```python
from build123d import *

# Parameters (mm, degrees)
CROQUIS1_W                 = 25.4
CROQUIS1_H                 = 25.4
SALIENTE_EXTRUIR1_DEPTH    = 40
SALIENTE_EXTRUIR3_DEPTH    = 17.5
SALIENTE_EXTRUIR4_REACH    = 76.655
CROQUIS6_W                 = 10
CROQUIS6_H                 = 20
CROQUIS9_R                 = 3.25
CORTAR_EXTRUIR3_DEPTH      = 10
CORTAR_EXTRUIR4_START      = -2.5
CROQUIS10_W                = 6.5
CROQUIS10_H                = 6.5
CORTAR_EXTRUIR4_DEPTH      = 10
CORTAR_EXTRUIR1_DEPTH      = 67.880303528
CORTAR_EXTRUIR1_DEPTH_BACK = 67.880303528
CROQUIS7_R                 = 3.5
SALIENTE_EXTRUIR5_START    = 21
CROQUIS11_W                = 10
CROQUIS11_H                = 10
CROQUIS11_R                = 3.5
SALIENTE_EXTRUIR5_DEPTH    = 21
SALIENTE_EXTRUIR6_START    = -10
SALIENTE_EXTRUIR6_DEPTH    = 10


with BuildPart() as part:
    # Croquis1 → Saliente-Extruir1 (new body)
    with BuildSketch(Plane(origin=(0, 0, 0), x_dir=(1, 0, 0), z_dir=(0, 1, 0))):
        Rectangle(CROQUIS1_W, CROQUIS1_H)
        Polygon((-10.2, 10.2), (-2.5, 10.2), (-2.5, 5.2), (2.5, 5.2), (2.5, 10.2), (10.2, 10.2), (10.2, 2.5), (5.2, 2.5), (5.2, -2.5), (10.2, -2.5), (10.2, -10.2), (2.5, -10.2), (2.5, -5.2), (-2.5, -5.2), (-2.5, -10.2), (-10.2, -10.2), (-10.2, -2.5), (-5.2, -2.5), (-5.2, 2.5), (-10.2, 2.5), align=None, mode=Mode.SUBTRACT)
    extrude(amount=SALIENTE_EXTRUIR1_DEPTH)



with BuildPart() as body_2:
    # Croquis4 → Saliente-Extruir3 (new, symmetric)
    with BuildSketch(Plane.XY):
        Polygon((-52.043145751, 35.556349186), (-47.093398282, 30.606601718), (-68.306601718, 9.393398282), (-73.256349186, 14.343145751), align=None)
    extrude(amount=SALIENTE_EXTRUIR3_DEPTH, both=True)


with BuildPart() as part_1:
    add(part.part)

    add(body_2.part)  # Saliente-Extruir4 merges body 2
    # Saliente-Extruir4: up to this plane
    saliente_extruir4_end = Plane(origin=(-68.306601718, 9.393398282, 17.5), z_dir=(-0.7071067811865436, 0.7071067811865516, 0))
    # Croquis6 → Saliente-Extruir4 (add, up to the surface)
    with BuildSketch(Plane.ZY.offset(12.7), mode=Mode.PRIVATE) as saliente_extruir4_sk1:
        with Locations((0, 20)):
            Rectangle(CROQUIS6_W, CROQUIS6_H)
    saliente_extruir4_tool1 = split(extrude(saliente_extruir4_sk1.sketch, amount=SALIENTE_EXTRUIR4_REACH, mode=Mode.PRIVATE), bisect_by=saliente_extruir4_end, keep=Keep.BOTH, mode=Mode.PRIVATE)
    add(saliente_extruir4_tool1.solids().sort_by_distance((-12.7, 20, 0))[0])

    # Croquis9 → Cortar-Extruir3 (cut)
    with BuildSketch(Plane(origin=(12.7, 0, 0), x_dir=(0, 0, -1), z_dir=(1, 0, 0))):
        with Locations((0, 20)):
            Circle(CROQUIS9_R)
    extrude(amount=-CORTAR_EXTRUIR3_DEPTH, mode=Mode.SUBTRACT)

    # Croquis10 → Cortar-Extruir4 (cut)
    with BuildSketch(Plane(origin=(12.7, 0, 0), x_dir=(0, 0, -1), z_dir=(1, 0, 0)).offset(CORTAR_EXTRUIR4_START)):
        with Locations((0, 20)):
            Rectangle(CROQUIS10_W, CROQUIS10_H)
    extrude(amount=-CORTAR_EXTRUIR4_DEPTH, mode=Mode.SUBTRACT)

    # Croquis7 → Cortar-Extruir1 (cut, two sides: drawn at the far end of the back side and taken through both)
    with BuildSketch(Plane(origin=(-38.85, 38.85, 0), x_dir=(0, 0, -1), z_dir=(0.7071067811865438, -0.7071067811865512, 0)).offset(-CORTAR_EXTRUIR1_DEPTH_BACK)):
        with Locations(Location((0, -26.657925651, 0), (0, 0, 90))):
            Circle(CROQUIS7_R)
    extrude(amount=CORTAR_EXTRUIR1_DEPTH + CORTAR_EXTRUIR1_DEPTH_BACK, mode=Mode.SUBTRACT)

    # Croquis11 → Saliente-Extruir5 (add)
    with BuildSketch(Plane(origin=(-38.85, 38.85, 0), x_dir=(0, 0, -1), z_dir=(0.7071067811865437, -0.7071067811865515, 0)).offset(SALIENTE_EXTRUIR5_START)):
        with Locations((0, -26.657925651)):
            Rectangle(CROQUIS11_W, CROQUIS11_H)
        with Locations(Location((0, -26.657925651, 0), (0, 0, 90))):
            Circle(CROQUIS11_R, mode=Mode.SUBTRACT)
    extrude(amount=-SALIENTE_EXTRUIR5_DEPTH)

    # Croquis12 → Saliente-Extruir6 (add)
    with BuildSketch(Plane.XY.offset(5).offset(SALIENTE_EXTRUIR6_START)):
        Polygon((-38.00151519, 10), (-40.628932188, 10), (-39.315223689, 8.686291501), align=None)
    extrude(amount=SALIENTE_EXTRUIR6_DEPTH)


solid = part_1.part
```
Source: CAD feature listing. Evaluate the final solid. Frame: model axes, mm. A direction names the side the tool comes from. Coordinates: 2 decimals unless noted, no trailing zeros. Write each loop counter-clockwise with the first axis right and the second up, starting at its lowest first coordinate (ties: lowest second). Pieces come first, ordered by that corner, then holes. Notation, with made-up numbers: M 23,88 L 77,88 A16 cw 77,105 Z; hole C 87,3 d8. An arc over 180 degrees is marked long. Answer as a JSON object with one key per item and string values.
1. Cut plane C-C on x = -23. Output: boundary loops of the cut face in (y, z).
Evaluation:
{"outline": "M 10,-5 L 30,-5 L 30,5 L 10,5 Z"}
2. Contact query for flat-ended pins moving along their axis: P1, Ø2, axis at x = -6.5, y = 22.5, coming from the +Z side; P2, Ø1.5, axis at x = 0.5, y = 10.5, coming from the -Z side; P3, Ø2.5, axis at y = 29.5, z = 1, coming from the -X side; P4, Ø10, axis at x = -31, z = -12, coming from the +Y side. Output: stop coordinate, or through.
Evaluation:
{"P1": "z = 12.7", "P2": "z = -12.7", "P3": "x = -59.35", "P4": "through"}
3. Cut plane A-A on z = 8.5. Output: boundary loops of the cut face in (x, y).
Evaluation:
{"outline": "M -73.26,14.34 L -68.31,9.39 L -47.09,30.61 L -52.04,35.56 Z; M -12.7,0 L -10.2,0 L -10.2,40 L -12.7,40 Z; M -2.5,0 L 2.5,0 L 2.5,40 L -2.5,40 Z; M 10.2,0 L 12.7,0 L 12.7,40 L 10.2,40 Z"}
4. Cut plane D-D on z = 1.5. State how many separate pieces and enclosed holes the cut face has, plus the area to 3 significant figures.
Evaluation:
{"separate pieces": "4", "enclosed holes": "0", "area": "1,560 mm^2"}
5. Access query for faces 1 (the flat face through (-62.8, 24.8, 4.1)), 2 (the flat face through (-61, 22, -17.5)), 3 (the flat face through (8, 23.25, 0)), 4 (the flat face through (-40, 8, -1)), 5 (the flat face through (-2.5, 20, 8)). Directions: +Z, -Z, +X, -X, +Y, -Y. A direction counts if a zero-diameter tool reaches every point of the face in a straight line with its end or side. Return the directions, or none.
Evaluation:
{"face 1": "+Z, -Z, -X, +Y", "face 2": "-Z, +X, -X, +Y, -Y", "face 3": "none", "face 4": "+Z, -Z, -Y", "face 5": "+Y, -Y"}
6. Ray query, L1, parallel to Z at x = 10.75, y = 20; L2, parallel to Y at x = 11.65, z = 0; L3, parallel to Z at x = -1.5, y = 19. Return the intervals inside material, ascending.
Evaluation:
{"L1": "-12.7 to -3.25, 3.25 to 12.7", "L2": "0 to 16.75, 23.25 to 40", "L3": "-12.7 to -5.2, 5.2 to 12.7"}
7. Cut plane B-B on y = 32.5. Output: boundary loops of the cut face in (x, z).
Evaluation:
{"outline": "M -55.1,-17.5 L -48.99,-17.5 L -48.99,17.5 L -55.1,17.5 Z; M -12.7,-12.7 L 12.7,-12.7 L 12.7,12.7 L -12.7,12.7 Z; hole M -10.2,-10.2 L -2.5,-10.2 L -2.5,-5.2 L 2.5,-5.2 L 2.5,-10.2 L 10.2,-10.2 L 10.2,-2.5 L 5.2,-2.5 L 5.2,2.5 L 10.2,2.5 L 10.2,10.2 L 2.5,10.2 L 2.5,5.2 L -2.5,5.2 L -2.5,10.2 L -10.2,10.2 L -10.2,2.5 L -5.2,2.5 L -5.2,-2.5 L -10.2,-2.5 Z"}
8. Draft query along Z for faces 6 (the flat face through (5.5, 0, -0.2)), 7 (the flat face through (-8, 20, 2.5)), 8 (the flat face through (-34, 19, -5)), 9 (the flat face through (0, 20, 12.7)). Return one class per face: released by +Z, released by -Z, zero draft, split by the parting line, or undercut.
Evaluation:
{"face 6": "zero draft", "face 7": "undercut", "face 8": "released by -Z", "face 9": "released by +Z"}
